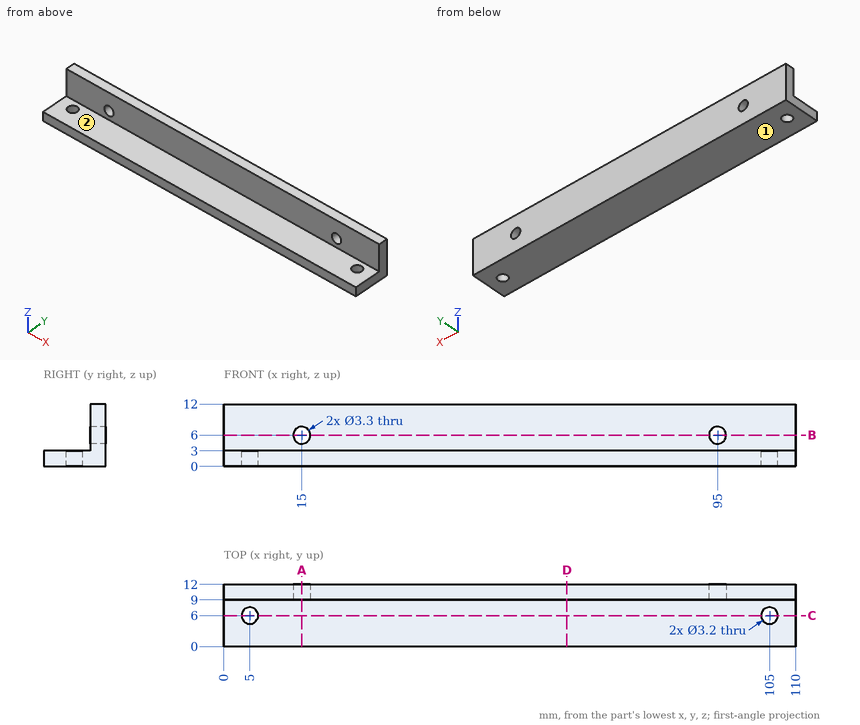
Input: dimensioned drawing with shaded views. Units: mm. Origin: part minimum x, y, z. A direction names the side the tool comes from. Coordinates: 2 decimals unless noted, no trailing zeros. Loops run counter-clockwise (first coordinate to the right, second up) from the corner with the lowest first, then second, coordinate; pieces in that order, holes last. Notation, with made-up numbers: M 56.5,6 L 66.5,6 A13 ccw 66.5,13 Z; hole C 29.25,86 d4. An arc over 180 degrees is marked long. Put each result on its own line as item: value.
(1) Material intervals for probe 1 along X at (y, z) = (6, 1.3); probe 2 along Z at (x, y) = (95, 10.2); probe 3 along X at (y, z) = (9.5, 5.5), sorted ascending.
Answer sheet:
probe 1: x = 0 to 3.4, 6.6 to 103.4, 106.6 to 110
probe 2: z = 0 to 4.35, 7.65 to 12
probe 3: x = 0 to 13.43, 16.57 to 93.43, 96.57 to 110
(2) Cut plane C-C on y = 6. Return the cut outline in (x, z), then the cut area to 3 significant figures.
Answer sheet:
outline: M 0,0 L 3.4,0 L 3.4,3 L 0,3 Z; M 6.6,0 L 103.4,0 L 103.4,3 L 6.6,3 Z; M 106.6,0 L 110,0 L 110,3 L 106.6,3 Z
area: 311 mm^2
(3) Access query for the marked faces 1 and 2. Directions: +Z, -Z, +X, -X, +Y, -Y. A direction counts if a zero-diameter tool reaches every point of the face in a straight line with its end or side. Return the directions, or none.
Answer sheet:
face 1: -Z, +X, -X, +Y, -Y
face 2: +Z, +X, -X, -Y
(4) Cut plane A-A on x = 15. Return the cut outline in (y, z).
Answer sheet:
outline: M 0,0 L 12,0 L 12,4.35 L 9,4.35 L 9,3 L 0,3 Z; M 9,7.65 L 12,7.65 L 12,12 L 9,12 Z
(5) First-contact query: pin 1 (1.9 mm diameter, centred on x = 5, y = 6, fed in from -Z); pin 2 (1.5 mm diameter, centred on x = 67.5, z = 9, fed in from -Y); pin 3 (4 mm diameter, centred on x = 74.5, y = 2, fed in from +Z). Flat tips, straight axial feed; report the tip coordinate or a pass-through.
Answer sheet:
pin 1: passes through
pin 2: stops at y = 9
pin 3: stops at z = 3
(6) Cut plane B-B on z = 6. Return the cut outline in (x, y).
Answer sheet:
outline: M 0,9 L 13.35,9 L 13.35,12 L 0,12 Z; M 16.65,9 L 93.35,9 L 93.35,12 L 16.65,12 Z; M 96.65,9 L 110,9 L 110,12 L 96.65,12 Z
(7) Cut plane D-D on x = 66. Return the cut outline in (y, z), then the cut area to 3 significant figures.
Answer sheet:
outline: M 0,0 L 12,0 L 12,12 L 9,12 L 9,3 L 0,3 Z
area: 63.0 mm^2
